For this review, take the finished solid that the model builds, in its own axes (mm). Round coordinates to 2 decimals unless told otherwise and drop trailing zeros. Loops run counter-clockwise (first coordinate to the right, second up) from the corner with the lowest first, then second, coordinate; pieces in that order, holes last. Notation, with made-up numbers: (-27, 70) -> (9, 70) arc R25 cw to (9, 88) -> close; hole circle Ø10 at (-28.75, 80). An arc over 180 degrees is marked (long way). Write each question's results on one line, items separated by ' | '.
```python
from build123d import *

# Parameters (mm, degrees)
F1_DEPTH = 3
F2_SIZE  = 1.49999


# Not quite as in the source:
# - a fillet or chamfer is up to 0.001 mm smaller than in the source, because OpenCascade refuses the exact size


with BuildPart() as f1:
    # F0 (on Front) → F1 (new body)
    with BuildSketch(Plane.XZ):
        with BuildLine():
            ThreePointArc((0, 0), (61.4781903769, -20.8298692006), (106.2082496532, -67.8689289283))
            ThreePointArc((106.2082496532, -67.8689289283), (73.6372514953, 2.0479582207), (0, 25))
            Line((0, 25), (0, 0))
        make_face()
    extrude(amount=F1_DEPTH)

    # F2 (size 1.5 in the source; OpenCascade refuses exactly that, so slightly less here)
    f2_edges = [f1.edges().sort_by_distance(p)[0] for p in [
        (73.637251, -3, 2.047958),
        (73.637251, 0, 2.047958),
    ]]
    chamfer(f2_edges, length=F2_SIZE)


solid = f1.part
```
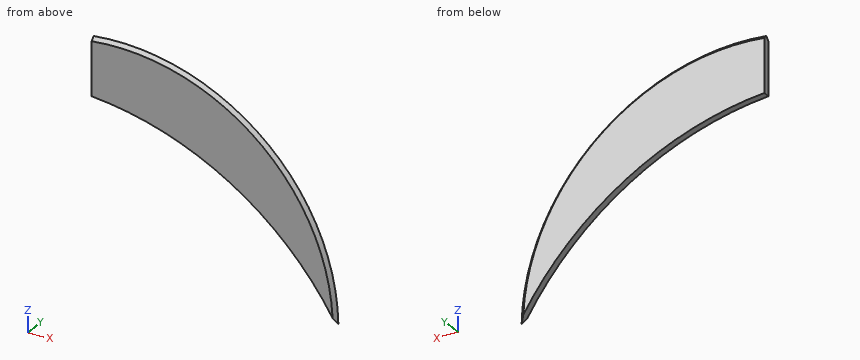
1. For pin 1 (12 mm diameter, centred on x = 90, z = 2.5, fed in from +Y); pin 2 (1 mm diameter, centred on x = 19.5, y = -2.5, fed in from -Z); pin 3 (1.5 mm diameter, centred on y = -2, z = -25.5, fed in from -X), all flat-tipped, find the tip position at first contact; note any pin that passes through.
Values found:
pin 1: passes through | pin 2: stops at z = -3.22 | pin 3: stops at x = 67.28
2. To check wall thickness, follow probe 1 along Z at (x, y) = (83.5, -0.9); probe 2 along Z at (x, y) = (25, -0.25); probe 3 along X at (y, z) = (-2.35, 2). State the ranges of each line that lie inside material, in increasing order.
Values found:
probe 1: z = -38.37 to -8.88 | probe 2: z = -4.51 to 23.3 | probe 3: x = 0 to 72.39
3. Consider section A-A (y = -0.55). State the section outline as (x, z) points, plus the area to 3 significant figures.
Values found:
outline: (0, 0) arc R135.47 cw to (105.21, -66.14) arc R94.41 ccw to (0, 24.04) -> close | area: 2,900 mm2
